from build123d import *

# Parameters (mm, degrees)
F1_DEPTH = 5
F2_W     = 17.85
F2_H     = 223.862902
F3_DEPTH = 4
F5_DEPTH = 3


with BuildPart() as f1:
    # F0 (on Front) → F1 (new body)
    with BuildSketch(Plane.XZ):
        Polygon((17.692703, 111.931451), (0, 111.931451), (0, -111.931451), (17.85, -111.931451), (23.26, -107.9006), (23.26, -94.031428), (17.85, -94.031428), (17.85, 94.281451), (20.929774, 96.176705), (20.929774, 98.249632), (23.26, 100.407617), (23.26, 106.389501), align=None)
    extrude(amount=F1_DEPTH)

    # F2 (on face) → F3 (join)
    with BuildSketch(Plane(origin=(0, 0, 0), x_dir=(-1, 0, 0), z_dir=(0, 1, 0))):
        with Locations((-8.925, 0)):
            Rectangle(F2_W, F2_H)
    extrude(amount=F3_DEPTH)


with BuildPart() as f5:
    # F4 (on face) → F5 (new body)
    with BuildSketch(Plane.XY.offset(111.931451)):
        with BuildLine():
            Line((6.925, -1), (7.510786, -1))
            ThreePointArc((7.510786, -1), (7.86434, -1.56066), (8.425, -1.914214))
            Line((8.425, -1.914214), (8.425, -2.5))
            Line((8.425, -2.5), (9.425, -2.5))
            Line((9.425, -2.5), (9.425, -1.914214))
            ThreePointArc((9.425, -1.914214), (9.98566, -1.56066), (10.339214, -1))
            Line((10.339214, -1), (10.925, -1))
            Line((10.925, -1), (10.925, 0))
            Line((10.925, 0), (10.339214, 0))
            ThreePointArc((10.339214, 0), (9.98566, 0.56066), (9.425, 0.914214))
            Line((9.425, 0.914214), (9.425, 1.5))
            Line((9.425, 1.5), (8.425, 1.5))
            Line((8.425, 1.5), (8.425, 0.914214))
            ThreePointArc((8.425, 0.914214), (7.86434, 0.56066), (7.510786, 0))
            Line((7.510786, 0), (6.925, 0))
            Line((6.925, 0), (6.925, -1))
        make_face()
    extrude(amount=-F5_DEPTH)


with BuildPart() as f6_1:
    # F6: instance of F5
    add(f5.part.mirror(Plane.XY))


with BuildPart() as f1_1:
    add(f1.part)

    # F7: cut F5
    add(f5.part, mode=Mode.SUBTRACT)

    # F8: cut F6_1
    add(f6_1.part, mode=Mode.SUBTRACT)


solid = f1_1.part
The listing builds one solid part. Answer for the finished solid, in the listing's coordinates (mm). A direction names the side the tool comes from. Coordinates: 2 decimals unless noted, no trailing zeros. Write each loop counter-clockwise with the first axis right and the second up, starting at its lowest first coordinate (ties: lowest second). Pieces come first, ordered by that corner, then holes. Notation, with made-up numbers: (-19, 33.5) - (15, 33.5) arc R24 ccw to (15, 64.5) - close; hole circle Ø3 at (82, 26.25). An arc over 180 degrees is marked (long way). Put each result on its own line as item: value.
1. Determine the mould class of faces 1 (the face through (20, 0, 103)), 2 (the face through (9, 0, 108.931)), 3 (the face through (0, -1, -2)) for opening direction Y: pulls with the +Y half, pulls with the -Y half, needs draft (parallel to the pull), parting line crosses it, or undercut.
Answer sheet:
face 1: pulls with the +Y half
face 2: undercut
face 3: needs draft
2. Find the intervals of material crossed by line 1 along X through (y, z) = (-1.5, 94); line 2 along Z through (x, y) = (10, -1.25); line 3 along Z through (x, y) = (21.75, -4.25), in increasing order. Write a range as from..to.
Answer sheet:
line 1: x = 0..17.85
line 2: z = -108.93..108.93
line 3: z = -109.03..-94.03, 99.01..107.89
3. A tool of negligible diameter and unlimited length cuts with its end or side. For faces 4 (the face through (21, 0, -103)), 5 (the face through (23.26, -2, -101)), 6 (the face through (21, -2, -94.031)), 7 (the face through (9, 0, -108.931)), 8 (the face through (9, 4, 2)), from which of +Z, -Z, +X, -X, +Y, -Y can it reach the whole face along a straight path? Write none if from no direction.
Answer sheet:
face 4: +Z, -Z, +X, +Y
face 5: +Z, -Z, +X, +Y, -Y
face 6: +X, +Y, -Y
face 7: -Z
face 8: +Z, -Z, +X, -X, +Y
4. The part is cut by section A-A on z = -84. Give the vertices of the cut face in (x, y), plus the area to 3 significant figures.
Answer sheet:
outline: (0, -5) - (17.85, -5) - (17.85, 4) - (0, 4) - close
area: 161 mm^2
5. Flat-ended cylindrical pins translate along their axes: pin 1 Ø1.1 at (y, z) = (-0.5, -110.5) entering from +X; pin 2 Ø1 at (y, z) = (-2.5, 1) entering from -X; pin 3 Ø0.6 at (y, z) = (1, -110.5) entering from +X. Find the tip coordinate at first contact, or state that the pin passes through.
Answer sheet:
pin 1: stops at x = 20.51
pin 2: stops at x = 0
pin 3: stops at x = 17.85
